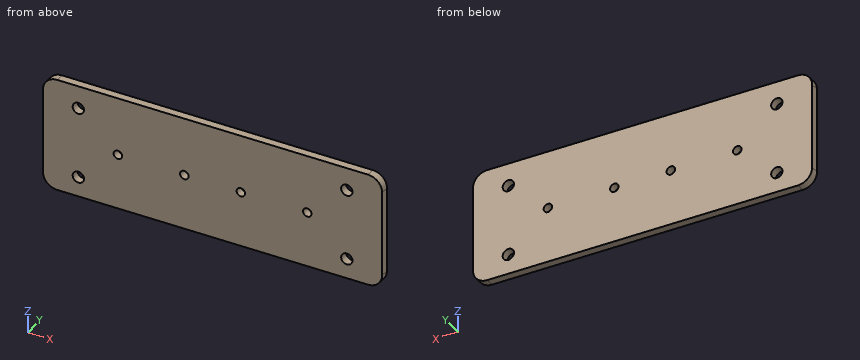
from build123d import *

# Parameters (mm, degrees)
SKETCH_1_W      = 120
SKETCH_1_H      = 40
SKETCH_1_R      = 1.5
SKETCH_1_R_2    = 2
EXTRUDE_1_DEPTH = 3
FILLET_1_R      = 5


with BuildPart() as part:
    # 草图1 → 凸台-拉伸1 (new body)
    with BuildSketch(Plane(origin=(0, 0, 0), x_dir=(1, 0, 0), z_dir=(0, 1, 0))):
        with Locations((0, 20)):
            Rectangle(SKETCH_1_W, SKETCH_1_H)
        with Locations(Location((10, 20.5, 0), (0, 0, 270))):
            Circle(SKETCH_1_R, mode=Mode.SUBTRACT)
        with Locations(Location((-10, 20.5, 0), (0, 0, 270))):
            Circle(SKETCH_1_R, mode=Mode.SUBTRACT)
        with Locations(Location((-33.5, 20.5, 0), (0, 0, 270))):
            Circle(SKETCH_1_R, mode=Mode.SUBTRACT)
        with Locations(Location((33.5, 20.5, 0), (0, 0, 270))):
            Circle(SKETCH_1_R, mode=Mode.SUBTRACT)
        with Locations(Location((-47.5, 8, 0), (0, 0, 270))):
            Circle(SKETCH_1_R_2, mode=Mode.SUBTRACT)
        with Locations(Location((-47.5, 33, 0), (0, 0, 270))):
            Circle(SKETCH_1_R_2, mode=Mode.SUBTRACT)
        with Locations(Location((47.5, 33, 0), (0, 0, 270))):
            Circle(SKETCH_1_R_2, mode=Mode.SUBTRACT)
        with Locations(Location((47.5, 8, 0), (0, 0, 270))):
            Circle(SKETCH_1_R_2, mode=Mode.SUBTRACT)
    extrude(amount=EXTRUDE_1_DEPTH)

    # 圆角1
    fillet_1_edges = [part.edges().sort_by_distance(p)[0] for p in [
        (-60, 1.5, -40),
        (60, 1.5, -40),
        (60, 1.5, 0),
        (-60, 1.5, 0),
    ]]
    fillet(fillet_1_edges, radius=FILLET_1_R)


solid = part.part
Model file for the job. Use its own axes, mm. Round coordinates to 2 decimals unless told otherwise and drop trailing zeros. Order: outer loops, then holes, each group sorted by start corner. A loop starts at its lowest first (then second) coordinate and runs counter-clockwise, first axis right, second up. Notation, with made-up numbers: M -13.5,40.5 L -9.5,40.5 A26 ccw -9.5,79.5 Z; hole C 79.25,-35 d1. An arc over 180 degrees is marked long. Write each question's results on one line, items separated by ' | '. Start each with the question number.
(1) Saw through at B-B, the plane x = 33.5. Give the cut face in (y, z).
(2) Saw through at A-A, the plane z = -8. Give the cut face in (x, y).
(3) Probe probe 1 along X at (y, z) = (1.7, -33); probe 2 along X at (y, z) = (1.8, -20.5); probe 3 along X at (y, z) = (2.05, -21). List the from-to ranges inside material, lowest first. Write a range as from..to.
(4) Drop a flat-ended pin along its axis: pin 1 (2.5 mm diameter, centred on x = -10, z = -20.5, fed in from +Y). Give the stop position or say it passes through.
(5) Saw through at C-C, the plane y = 0.9. State how many separate pieces and enclosed holes the cut face has, then the cut area to 3 significant figures.
(6) Saw through at D-D, the plane x = -47.5. Give the cut face in (y, z).
Established:
1) outline: M 0,-40 L 3,-40 L 3,-22 L 0,-22 Z; M 0,-19 L 3,-19 L 3,0 L 0,0 Z
2) outline: M -60,0 L -49.5,0 L -49.5,3 L -60,3 Z; M -45.5,0 L 45.5,0 L 45.5,3 L -45.5,3 Z; M 49.5,0 L 60,0 L 60,3 L 49.5,3 Z
3) probe 1: x = -60..-49.5, -45.5..45.5, 49.5..60 | probe 2: x = -60..-35, -32..-11.5, -8.5..8.5, 11.5..32, 35..60 | probe 3: x = -60..-34.91, -32.09..-11.41, -8.59..8.59, 11.41..32.09, 34.91..60
4) pin 1: passes through
5) separate pieces: 1 | enclosed holes: 8 | area: 4,700 mm^2
6) outline: M 0,-40 L 3,-40 L 3,-35 L 0,-35 Z; M 0,-31 L 3,-31 L 3,-10 L 0,-10 Z; M 0,-6 L 3,-6 L 3,0 L 0,0 Z
